Autodesk Inventor part; units mm, degrees
ref_plane "YZ Plane" through (0, 0, 0) normal (1, 0, 0) x (0, 1, 0)
ref_plane "XZ Plane" through (0, 0, 0) normal (0, 1, 0) x (-1, 0, 0)
ref_plane "XY Plane" through (0, 0, 0) normal (0, 0, 1) x (1, 0, 0)
sketch "Эскиз2" plane through (0, 0, 0) normal (0, 0, 1) x (1, 0, 0)
  line L0 (0, 0) -> (40.5, 0)
  line L1 (40.5, 0) -> (40.5, -20)
  line L2 (40.5, -20) -> (0, -20)
  line L3 (0, -20) -> (0, 0)
  line L4 (40.5, 0) -> (40.5, -4.7)
  line L5 (40.5, -4.7) -> (45.2, -4.7)
  line L6 (45.2, -15.3) -> (40.5, -15.3)
  line L7 (40.5, -15.3) -> (40.5, -20)
  line L8 (0, -4.7) -> (-4.7, -4.7)
  line L9 (-4.7, -15.3) -> (0, -15.3)
  line L10 (0, 0) -> (-7, 0)
  line L11 (-7, 0) -> (-7, -20)
  line L12 (-7, -20) -> (40.5, -20)
  line L13 (40.5, -20) -> (47.5, -20)
  line L14 (47.5, -20) -> (47.5, 0)
  line L15 (47.5, 0) -> (40.5, 0)
  circle A0 centre (-4.7, -4.7) radius 1.4
  circle A1 centre (-4.7, -15.3) radius 1.4
  circle A2 centre (45.2, -4.7) radius 1.4
  circle A3 centre (45.2, -15.3) radius 1.4
  dimension "d9" = 40.5
  dimension "d11" = 4.7
  dimension "d12" = 4.7
  dimension "d14" = 4.7
  dimension "d15" = 7
  dimension "d16" = 7
  dimension "d17" = 2.8
  dimension "d18" = 2.8
  dimension "d19" = 2.8
  dimension "d20" = 2.8
extrude "Выдавливание2" add sketch "Эскиз2" along normal blind 6 contours L3 L12 L11 L10 | L15 L14 L13 L1
sketch "Эскиз3" plane through (-7, -20, 0) normal (0, -1, 0) x (1, 0, 0)
  line L0 (7, 6) -> (0, 6)
  line L1 (47.5, 0) -> (54.5, 0)
  line L2 (0, 6) -> (54.5, 6)
  line L3 (54.5, 6) -> (54.5, 0)
  line L4 (54.5, 0) -> (0, 0)
  line L5 (0, 0) -> (0, 6)
  line L6 (47.5, 0) -> (47.5, 6)
  line L7 (47.5, 6) -> (37.5, 6)
  line L8 (37.5, 6) -> (54.0635, 6)
  line L9 (54.0635, 6) -> (20.9365, 6)
  line L10 (20.9365, 6) -> (20.9365, 1)
  line L11 (20.9365, 1) -> (54.0635, 1)
  line L12 (54.0635, 1) -> (54.0635, 6)
  circle A0 centre (20.9365, 1) radius 1.6
  circle A1 centre (54.0635, 1) radius 1.6
  line L13 (0, 6) -> (60, 6)
  line L14 (60, 6) -> (60, -4)
  line L15 (60, -4) -> (0, -4)
  line L16 (0, -4) -> (0, 6)
  point P0 (7, 0)
  point P1 (0, 0)
  dimension "d23" = 10
  dimension "d24" = 16.5635
  dimension "d25" = 33.127
  dimension "d26" = 5
  dimension "d27" = 3.2
  dimension "d28" = 3.2
  dimension "d29" = 60
  dimension "d30" = 10
extrude "Выдавливание3" add sketch "Эскиз3" along normal blind 6 contours L2 L10 A0 L4 L5 L0 | L2 L6 L11 A0 L10 | L4 A0 L1 A1 L3 L13 L14 L15 L16 | L2 L12 A1 L11 L6 | L11 L6 L4 A0 | L2 L3 A1 L12 | L11 A1 L1 L6
properties part number "vydacha_3"
Geometry: final body of the model. Coordinates: model frame, mm. A direction names the side the tool comes from. Round coordinates to 2 decimals unless told otherwise and drop trailing zeros. Loops run counter-clockwise (first coordinate to the right, second up) from the corner with the lowest first, then second, coordinate; pieces in that order, holes last. Notation, with made-up numbers: (-22.5, -28) - (32.5, -28) arc R33 cw to (32.5, 8) - close; hole circle Ø4 at (-1, 82). An arc over 180 degrees is marked (long way). Write each question's results on one line, items separated by ' | '. Start each with the question number.
1) Cut plane A-A on z = 1. Return loops of the section in (x, y), then the cut area to 3 significant figures.
2) Cut plane B-B on x = -4.7. Return loops of the section in (y, z), then the cut area to 3 significant figures.
3) Cut plane C-C on y = -4.7. Return loops of the section in (x, z), then the cut area to 3 significant figures.
4) Cut plane D-D on z = 4. Return loops of the section in (x, y).
5) Mould query, pull axis X, two halves, no side actions, for faces 4 (the face through (44, -10, 0)), 5 (the face through (23, -20, 1)), 6 (the face through (-7, -16, 2)). Classes: released by +X, released by -X, zero draft, split by the parting line, or undercut.
6) Line query: probe 1 along Y at (x, z) = (-4.7, 3.5); probe 2 along X at (y, z) = (-6.75, 4); probe 3 along Y at (x, z) = (7, -1.25). Output: solid intervals per line, ascending. Write a range as [from, to].
7) First-contact query: P1, Ø5.5, axis at x = 44.5, y = -6.5, coming from the -Z side; P2, Ø3, axis at y = -9, z = 4, coming from the +X side; P3, Ø5, axis at x = 43, z = -3, coming from the +Y side. Flat tips, straight axial feed; report the tip coordinate or a pass-through.
8) Access query for faces 1 (the face through (-4, -10, 0)), 2 (the face through (0, -10, 3)), 3 (the face through (46, -20, 1)). Directions: +Z, -Z, +X, -X, +Y, -Y. A direction counts if a zero-diameter tool reaches every point of the face in a straight line with its end or side. Return the directions, or none.
Verdict:
1) outline: (-7, -26) - (12.34, -26) - (12.34, -20) - (0, -20) - (0, 0) - (-7, 0) - close; (15.54, -26) - (45.46, -26) - (45.46, -20) - (47.5, -20) - (47.5, 0) - (40.5, 0) - (40.5, -20) - (15.54, -20) - close; (48.66, -26) - (53, -26) - (53, -20) - (48.66, -20) - close; hole circle Ø2.8 at (-4.7, -15.3); hole circle Ø2.8 at (-4.7, -4.7); hole circle Ø2.8 at (45.2, -15.3); hole circle Ø2.8 at (45.2, -4.7) | area: 577 mm2
2) outline: (-26, -4) - (-20, -4) - (-20, 0) - (-16.7, 0) - (-16.7, 6) - (-26, 6) - close; (-13.9, 0) - (-6.1, 0) - (-6.1, 6) - (-13.9, 6) - close; (-3.3, 0) - (0, 0) - (0, 6) - (-3.3, 6) - close | area: 146 mm2
3) outline: (-7, 0) - (-6.1, 0) - (-6.1, 6) - (-7, 6) - close; (-3.3, 0) - (0, 0) - (0, 6) - (-3.3, 6) - close; (40.5, 0) - (43.8, 0) - (43.8, 6) - (40.5, 6) - close; (46.6, 0) - (47.5, 0) - (47.5, 6) - (46.6, 6) - close | area: 50.4 mm2
4) outline: (-7, -26) - (53, -26) - (53, -20) - (47.5, -20) - (47.5, 0) - (40.5, 0) - (40.5, -20) - (0, -20) - (0, 0) - (-7, 0) - close; hole circle Ø2.8 at (-4.7, -15.3); hole circle Ø2.8 at (-4.7, -4.7); hole circle Ø2.8 at (45.2, -15.3); hole circle Ø2.8 at (45.2, -4.7)
5) face 4: zero draft | face 5: undercut | face 6: released by -X
6) probe 1: y = [-26, -16.7], [-13.9, -6.1], [-3.3, 0] | probe 2: x = [-7, 0], [40.5, 47.5] | probe 3: y = [-26, -20]
7) P1: stops at z = 0 | P2: stops at x = 47.5 | P3: stops at y = -20
8) face 1: -Z, +X, -X, +Y | face 2: +Z, -Z, +Y | face 3: -Y
